from build123d import *

# Parameters (mm, degrees)
F0_W      = 7.8
F0_H      = 15.8
F2_DEPTH  = 9.6
F3_R      = 2.45
F4_DEPTH  = 1.9
F6_DEPTH  = 8.3
F7_DEPTH  = 8.3
F8_DEPTH  = 8.3
F9_DEPTH  = 8.3
F10_DEPTH = 2
F11_DEPTH = 2


with BuildPart() as f2:
    # F0 (on Top) → F2 (new body)
    with BuildSketch(Plane.XY):
        with Locations((-57.467087, 32.808982)):
            Rectangle(F0_W, F0_H)
    extrude(amount=F2_DEPTH)

    # F3 (on face) → F4 (join)
    with BuildSketch(Plane.XY.offset(9.6)):
        with Locations((-57.467087, 36.758982)):
            Circle(F3_R)
        with Locations((-57.467087, 28.858982)):
            Circle(F3_R)
    extrude(amount=F4_DEPTH)

    # F5 (on face) → F6 (cut)
    with BuildSketch(Plane(origin=(0, 0, 0), x_dir=(1, 0, 0), z_dir=(0, 0, -1))):
        with BuildLine():
            Line((-55.067087, -26.408982), (-59.867087, -26.408982))
            Line((-59.867087, -26.408982), (-59.867087, -32.783981))
            Line((-59.867087, -32.783981), (-59.016885, -32.783981))
            ThreePointArc((-59.016885, -32.783981), (-57.467087, -31.258982), (-55.917289, -32.783981))
            Line((-55.917289, -32.783981), (-55.067087, -32.783981))
            Line((-55.067087, -32.783981), (-55.067087, -26.408982))
        make_face()
    extrude(amount=-F6_DEPTH, mode=Mode.SUBTRACT)

    # F5 (on face) → F7 (cut)
    with BuildSketch(Plane(origin=(0, 0, 0), x_dir=(1, 0, 0), z_dir=(0, 0, -1))):
        with BuildLine():
            Line((-55.067087, -26.408982), (-59.867087, -26.408982))
            Line((-59.867087, -26.408982), (-59.867087, -32.783981))
            Line((-59.867087, -32.783981), (-59.016885, -32.783981))
            ThreePointArc((-59.016885, -32.783981), (-57.467087, -31.258982), (-55.917289, -32.783981))
            Line((-55.917289, -32.783981), (-55.067087, -32.783981))
            Line((-55.067087, -32.783981), (-55.067087, -26.408982))
        make_face()
        with BuildLine():
            Line((-59.016885, -32.783981), (-59.867087, -32.783981))
            Line((-59.867087, -32.783981), (-59.867087, -32.833982))
            Line((-59.867087, -32.833982), (-59.016885, -32.833982))
            ThreePointArc((-59.016885, -32.833982), (-59.017087, -32.808982), (-59.016885, -32.783981))
        make_face()
        with BuildLine():
            Line((-55.067087, -32.833982), (-55.067087, -32.783981))
            Line((-55.067087, -32.783981), (-55.917289, -32.783981))
            ThreePointArc((-55.917289, -32.783981), (-55.917137, -32.796481), (-55.917087, -32.808982))
            ThreePointArc((-55.917087, -32.808982), (-55.917137, -32.821483), (-55.917289, -32.833982))
            Line((-55.917289, -32.833982), (-55.067087, -32.833982))
        make_face()
        with BuildLine():
            Line((-59.016885, -32.833982), (-59.867087, -32.833982))
            Line((-59.867087, -32.833982), (-59.867087, -39.208982))
            Line((-59.867087, -39.208982), (-55.067087, -39.208982))
            Line((-55.067087, -39.208982), (-55.067087, -32.833982))
            Line((-55.067087, -32.833982), (-55.917289, -32.833982))
            ThreePointArc((-55.917289, -32.833982), (-57.467087, -34.358982), (-59.016885, -32.833982))
        make_face()
    extrude(amount=-F7_DEPTH, mode=Mode.SUBTRACT)

    # F5 (on face) → F8 (join)
    with BuildSketch(Plane(origin=(0, 0, 0), x_dir=(1, 0, 0), z_dir=(0, 0, -1))):
        with BuildLine():
            Line((-55.067087, -32.833982), (-55.067087, -32.783981))
            Line((-55.067087, -32.783981), (-55.917289, -32.783981))
            ThreePointArc((-55.917289, -32.783981), (-55.917137, -32.796481), (-55.917087, -32.808982))
            ThreePointArc((-55.917087, -32.808982), (-55.917137, -32.821483), (-55.917289, -32.833982))
            Line((-55.917289, -32.833982), (-55.067087, -32.833982))
        make_face()
    extrude(amount=-F8_DEPTH)

    # F5 (on face) → F9 (join)
    with BuildSketch(Plane(origin=(0, 0, 0), x_dir=(1, 0, 0), z_dir=(0, 0, -1))):
        with BuildLine():
            Line((-59.016885, -32.783981), (-59.867087, -32.783981))
            Line((-59.867087, -32.783981), (-59.867087, -32.833982))
            Line((-59.867087, -32.833982), (-59.016885, -32.833982))
            ThreePointArc((-59.016885, -32.833982), (-59.017087, -32.808982), (-59.016885, -32.783981))
        make_face()
    extrude(amount=-F9_DEPTH)

    # F5 (on face) → F10 (cut)
    with BuildSketch(Plane(origin=(0, 0, 0), x_dir=(1, 0, 0), z_dir=(0, 0, -1))):
        with BuildLine():
            Line((-59.016885, -32.783981), (-59.867087, -32.783981))
            Line((-59.867087, -32.783981), (-59.867087, -32.833982))
            Line((-59.867087, -32.833982), (-59.016885, -32.833982))
            ThreePointArc((-59.016885, -32.833982), (-59.017087, -32.808982), (-59.016885, -32.783981))
        make_face()
    extrude(amount=-F10_DEPTH, mode=Mode.SUBTRACT)

    # F5 (on face) → F11 (cut)
    with BuildSketch(Plane(origin=(0, 0, 0), x_dir=(1, 0, 0), z_dir=(0, 0, -1))):
        with BuildLine():
            Line((-55.067087, -32.833982), (-55.067087, -32.783981))
            Line((-55.067087, -32.783981), (-55.917289, -32.783981))
            ThreePointArc((-55.917289, -32.783981), (-55.917137, -32.796481), (-55.917087, -32.808982))
            ThreePointArc((-55.917087, -32.808982), (-55.917137, -32.821483), (-55.917289, -32.833982))
            Line((-55.917289, -32.833982), (-55.067087, -32.833982))
        make_face()
    extrude(amount=-F11_DEPTH, mode=Mode.SUBTRACT)


solid = f2.part
Build history of the part. All positions in model axes, mm. A direction names the side the tool comes from. Round coordinates to 2 decimals unless told otherwise and drop trailing zeros. Write each loop counter-clockwise with the first axis right and the second up, starting at its lowest first coordinate (ties: lowest second). Pieces come first, ordered by that corner, then holes. Notation, with made-up numbers: M 52,45.25 L 88,45.25 A21 cw 88,53.25 Z; hole C -36,2 d5. An arc over 180 degrees is marked long. Answer in a Markdown table with one row per item.
1. Saw through at B-B (y = 29.5). List the corners of the cut face in (x, z).
Geometry check:
| item | result |
|---|---|
| outline | M -61.37,0 L -59.87,0 L -59.87,8.3 L -55.07,8.3 L -55.07,0 L -53.57,0 L -53.57,9.6 L -55.1,9.6 L -55.1,11.5 L -59.83,11.5 L -59.83,9.6 L -61.37,9.6 Z |
2. Saw through at C-C (x = -58.75). List the corners of the cut face in (y, z), and give its area (3 significant figures).
Geometry check:
| item | result |
|---|---|
| outline | M 24.91,0 L 26.41,0 L 26.41,8.3 L 31.94,8.3 L 31.94,0 L 33.68,0 L 33.68,8.3 L 39.21,8.3 L 39.21,0 L 40.71,0 L 40.71,9.6 L 38.85,9.6 L 38.85,11.5 L 34.67,11.5 L 34.67,9.6 L 30.95,9.6 L 30.95,11.5 L 26.77,11.5 L 26.77,9.6 L 24.91,9.6 Z |
| area | 75.7 mm2 |
3. Flat gauge pin, fed straight in: P1, Ø2.5, axis at x = -58.5, y = 37.5, coming from the -Z side. Where does the tip first touch, or does it go through?
Geometry check:
| item | result |
|---|---|
| P1 | z = 8.3 |
4. Which spindle directions (+Z, -Z, +X, -X, +Y, -Y) get a long thin tool onto all of the face, cutting with end or side? Do faces 4 (the face through (-55.067, 33, 4)), 5 (the face through (-58, 33, 9.6)), 6 (the face through (-61.367, 33, 5)). Say none if no direction does.
Geometry check:
| item | result |
|---|---|
| face 4 | -Z |
| face 5 | +Z |
| face 6 | +Z, -Z, -X, +Y, -Y |
5. Saw through at D-D (y = 34). List the corners of the cut face in (x, z).
Geometry check:
| item | result |
|---|---|
| outline | M -61.37,0 L -59.87,0 L -59.87,8.3 L -58.46,8.3 L -58.46,0 L -56.48,0 L -56.48,8.3 L -55.07,8.3 L -55.07,0 L -53.57,0 L -53.57,9.6 L -61.37,9.6 Z |
6. Saw through at A-A (z = 6.25). List the corners of the cut face in (x, y), and give its area (3 significant figures).
Geometry check:
| item | result |
|---|---|
| outline | M -61.37,24.91 L -53.57,24.91 L -53.57,40.71 L -61.37,40.71 Z; hole M -59.87,26.41 L -55.07,26.41 L -55.07,32.78 L -55.92,32.78 A1.55 cw -59.02,32.78 L -59.87,32.78 Z; hole M -59.87,32.83 L -59.02,32.83 A1.55 cw -55.92,32.83 L -55.07,32.83 L -55.07,39.21 L -59.87,39.21 Z |
| area | 69.4 mm2 |
7. Probe L1, parallel to X at y = 36.75, z = 5; L2, parallel to Y at x = -57, z = 2.25; L3, parallel to Y at x = -58.25, z = 5.75. List the from-to ranges inside material, lowest first. Write a range as [from, to].
Geometry check:
| item | result |
|---|---|
| L1 | [-61.37, -59.87], [-55.07, -53.57] |
| L2 | [24.91, 26.41], [31.33, 34.29], [39.21, 40.71] |
| L3 | [24.91, 26.41], [31.47, 34.15], [39.21, 40.71] |
8. Mould opens along Y. For faces 1 (the face through (-54.9, 32.7, 0)), 2 (the face through (-58, 30, 8.3)), 3 (the face through (-58, 40.709, 5)) say: +Y half, -Y half, draft (parallel to the pull), parting line (faces both ways), or undercut.
Geometry check:
| item | result |
|---|---|
| face 1 | draft |
| face 2 | undercut |
| face 3 | +Y half |
